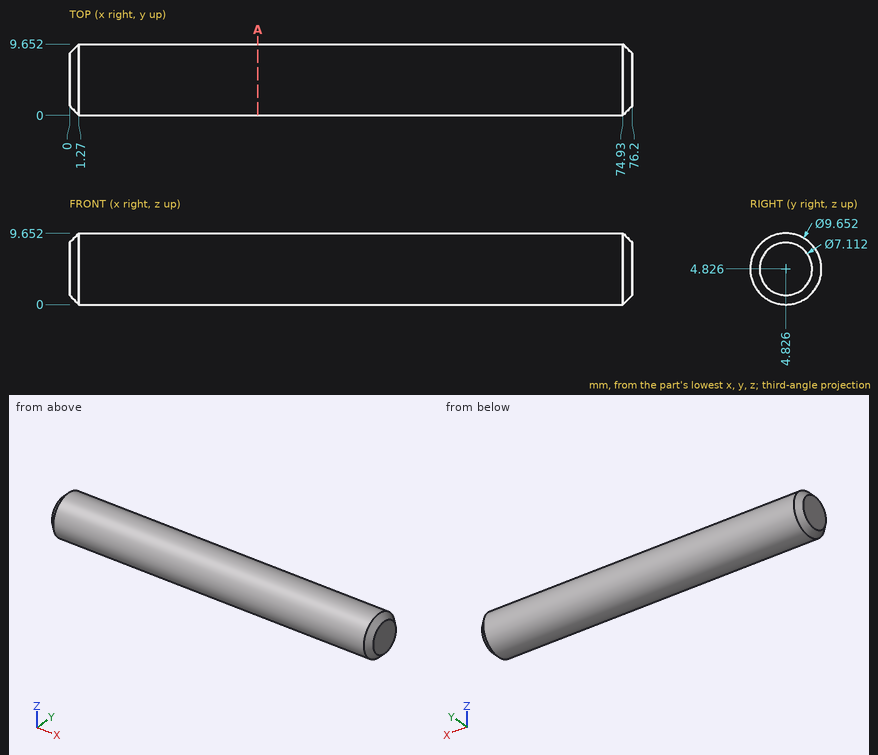
Verification items for this drawing (mm, ordinates from the low corner). Coordinates: 2 decimals unless noted, no trailing zeros. Write each loop counter-clockwise with the first axis right and the second up, starting at its lowest first coordinate (ties: lowest second). Pieces come first, ordered by that corner, then holes. Notation, with made-up numbers: M -11,43 L -1,43 A4 cw -1,50 Z; hole C 48.25,40.5 d1. An arc over 180 degrees is marked long. One line per item, written item: value. Start each with the question number.
(1) Scan lines: line 1 along Z through (x, y) = (16.5, 7); line 2 along Z through (x, y) = (38, 1.5); line 3 along Y through (x, z) = (58, 0.5). Record each from-to range of solid material in increasing order. Write a range as [from, to].
(2) Sectioned sample at A-A, the plane x = 25.5. Enter the section's corners in (y, z), and give its area (3 significant figures).
(3) Depth check by flat-ended pin: pin 1 (1.5 mm diameter, centred on x = 15.5, y = 8, fed in from -Z); pin 2 (3 mm diameter, centred on x = 44.5, z = 8, fed in from +Y). Enter the tip coordinate at first touch or a pass-through.
Filled sheet:
1. line 1: [0.52, 9.13]
1. line 2: [1.33, 8.32]
1. line 3: [2.69, 6.97]
2. outline: C 4.83,4.83 d9.65
2. area: 73.2 mm²
3. pin 1: z = 0.65
3. pin 2: y = 9.35
